Read the model definition and answer for the solid it produces. Units are mm, in the model's axes. A direction names the side the tool comes from. Round coordinates to 2 decimals unless told otherwise and drop trailing zeros. Write each loop counter-clockwise with the first axis right and the second up, starting at its lowest first coordinate (ties: lowest second). Pieces come first, ordered by that corner, then holes. Notation, with made-up numbers: (8.5, 51) - (29.5, 51) arc R19 cw to (29.5, 60) - close; hole circle Ø10 at (50, -6). An arc over 180 degrees is marked (long way). Use one line per item in the form item = value. Start each with the question number.
1) The part is cut by section D-D, the plane x = -5.25. Give the vertices of the cut face in (y, z), plus the area to 3 significant figures.
2) Consider line 1 along Y through (x, z) = (0, 18); line 2 along Z through (x, y) = (0, -446); line 3 along Y through (x, z) = (9, 20.5). Determine where each line is inside the solid, lowest interval first. Write a range as from..to.
3) The part is cut by section C-C, the plane y = -446.5. Give the vertices of the cut face in (x, z), plus the area to 3 significant figures.
4) For a pull along X with two mould halves and no side action, classify faces 3 (the face through (1.846, -477.549, 18.14)), 4 (the face through (3, -439, 16)), 5 (the face through (-0.976, -444.916, 25.436)) as released by +X, released by -X, zero draft, split by the parting line, or undercut.
5) For faces 1 (the face through (-0.683, -444.916, 14.925)), 2 (the face through (0, -481, 18)), determine the directions among +Z, -Z, +X, -X, +Y, -Y from which every point of the face is accessible in a straight line to the end or side of a thin tool.
6) Each of these flat-tipped pins is pushed along its axis until it touches: pin 1 (7 mm diameter, centred on x = -1, z = 18, fed in from +Y); pin 2 (3 mm diameter, centred on x = -2.5, y = -446.5, fed in from -Z); pin 3 (4 mm diameter, centred on x = 6.5, y = -475, fed in from -Z); pin 4 (4 mm diameter, centred on x = 1.5, y = -476, fed in from +Z). Where does it stop, or does it pass through?
7) The part is cut by section B-B, the plane x = 0. Give the vertices of the cut face in (y, z).
8) The part is cut by section A-A, the plane z = 18. Give the vertices of the cut face in (x, y).
from build123d import *

# Parameters (mm, degrees)
SKETCH004_R       = 7.5
SKETCH004_R_2     = 3.15
PAD004_DEPTH      = 12
SKETCH005_R       = 10
PAD005_DEPTH      = 30
SKETCH006_R       = 4
POCKET_DEPTH      = 10.001
POCKET_DEPTH_BACK = 10.001


with BuildPart() as part:
    # Sketch004 → Pad004 (new body)
    with BuildSketch(Plane.XZ):
        Circle(SKETCH004_R)
        Circle(SKETCH004_R_2, mode=Mode.SUBTRACT)
    extrude(amount=PAD004_DEPTH)

    # Sketch005 → Pad005 (join)
    with BuildSketch(Plane.XZ.offset(12)):
        Circle(SKETCH005_R)
    extrude(amount=PAD005_DEPTH)

    # Sketch006 → Pocket (cut, two sides)
    with BuildSketch(Plane(origin=(0, -35, 0), x_dir=(1, 0, 0), z_dir=(0, 0, 1))) as pocket_sk:
        Circle(SKETCH006_R)
    extrude(amount=-POCKET_DEPTH, mode=Mode.SUBTRACT)
    extrude(pocket_sk.sketch, amount=POCKET_DEPTH_BACK, mode=Mode.SUBTRACT)


with BuildPart() as part_1:
    # Body002 placement: moved
    add(part.part.moved(Location((0, -439, 18))))


solid = part_1.part
Geometry results:
q1.outline = (-481, 9.49) - (-451, 9.49) - (-451, 12.64) - (-439, 12.64) - (-439, 23.36) - (-451, 23.36) - (-451, 26.51) - (-481, 26.51) - close
q1.area = 639 mm2
q2.line_1 = -481..-478, -470..-451
q2.line_2 = 10.5..14.85, 21.15..25.5
q2.line_3 = -481..-451
q3.outline = circle Ø15 at (0, 18); hole circle Ø6.3 at (0, 18)
q3.area = 146 mm2
q4.face_3 = undercut
q4.face_4 = zero draft
q4.face_5 = split by the parting line
q5.face_1 = +Y
q5.face_2 = +Z, -Z, +X, -X, -Y
q6.pin_1 = -439
q6.pin_2 = 10.57
q6.pin_3 = 9.07
q6.pin_4 = 27.96
q7.outline = (-481, 8) - (-478, 8) - (-478, 28) - (-481, 28) - close; (-470, 8) - (-451, 8) - (-451, 10.5) - (-439, 10.5) - (-439, 14.85) - (-451, 14.85) - (-451, 21.15) - (-439, 21.15) - (-439, 25.5) - (-451, 25.5) - (-451, 28) - (-470, 28) - close
q8.outline = (-10, -481) - (10, -481) - (10, -451) - (7.5, -451) - (7.5, -439) - (3.15, -439) - (3.15, -451) - (-3.15, -451) - (-3.15, -439) - (-7.5, -439) - (-7.5, -451) - (-10, -451) - close; hole circle Ø8 at (0, -474)
